Part print with two shaded views. Sizes in mm from the minimum x, y, z corner. Round coordinates to 2 decimals unless told otherwise and drop trailing zeros. Write each loop counter-clockwise with the first axis right and the second up, starting at its lowest first coordinate (ties: lowest second). Pieces come first, ordered by that corner, then holes. Notation, with made-up numbers: (-32.5, 76) -> (23.5, 76) arc R21 ccw to (23.5, 87) -> close; hole circle Ø11 at (57.5, -22.75). An arc over 180 degrees is marked (long way). Answer in a Markdown table with one row per item.
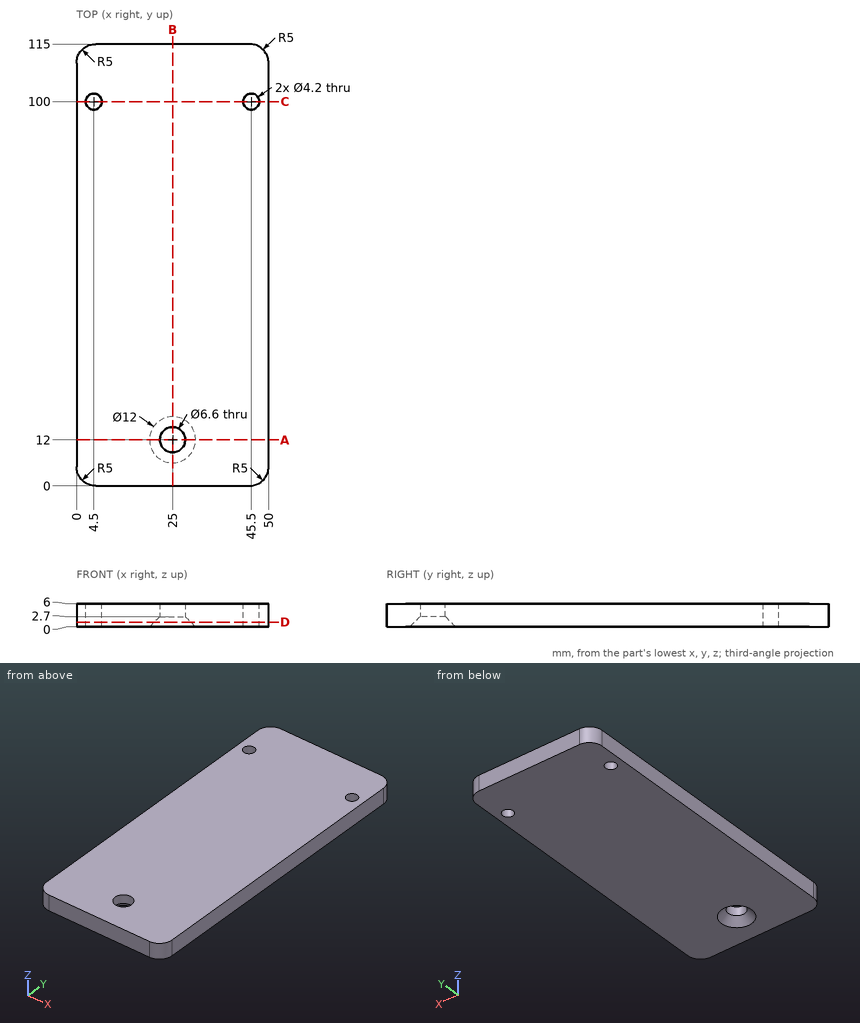
Q1. Saw through at B-B on x = 25. Write the cut outline in (y, z).
A:
| item | result |
|---|---|
| outline | (0, 0) -> (6, 0) -> (8.7, 2.7) -> (8.7, 6) -> (0, 6) -> close; (15.3, 2.7) -> (18, 0) -> (115, 0) -> (115, 6) -> (15.3, 6) -> close |
Q2. Saw through at A-A on y = 12. Write the cut outline in (x, z).
A:
| item | result |
|---|---|
| outline | (0, 0) -> (19, 0) -> (21.7, 2.7) -> (21.7, 6) -> (0, 6) -> close; (28.3, 2.7) -> (31, 0) -> (50, 0) -> (50, 6) -> (28.3, 6) -> close |
Q3. Saw through at D-D on z = 1.25. Write the cut outline in (x, y).
A:
| item | result |
|---|---|
| outline | (0, 5) arc R5 ccw to (5, 0) -> (45, 0) arc R5 ccw to (50, 5) -> (50, 110) arc R5 ccw to (45, 115) -> (5, 115) arc R5 ccw to (0, 110) -> close; hole circle Ø4.2 at (4.5, 100); hole circle Ø9.5 at (25, 12); hole circle Ø4.2 at (45.5, 100) |
Q4. Wall check: line 1 (Y direction, x = 45.5, z = 2); line 2 (X direction, y = 100, z = 3.2); line 3 (X direction, y = 9, z = 2.2). Give the ranges that are in metal, low to high. Write a range as [from, to].
A:
| item | result |
|---|---|
| line 1 | [0.03, 97.9], [102.1, 114.97] |
| line 2 | [0, 2.4], [6.6, 43.4], [47.6, 50] |
| line 3 | [0, 22.67], [27.33, 50] |
Q5. Saw through at C-C on y = 100. Write the cut outline in (x, z), plus the area to 3 significant figures.
A:
| item | result |
|---|---|
| outline | (0, 0) -> (2.4, 0) -> (2.4, 6) -> (0, 6) -> close; (6.6, 0) -> (43.4, 0) -> (43.4, 6) -> (6.6, 6) -> close; (47.6, 0) -> (50, 0) -> (50, 6) -> (47.6, 6) -> close |
| area | 250 mm² |
